from build123d import *

# Parameters (mm, degrees)
F0_W      = 100
F0_H      = 70
F1_DEPTH  = 60
F3_DEPTH  = 70.001
F4_R      = 2
F5_DEPTH  = 60.001
F6_R      = 28.75
F7_DEPTH  = 60.001
F8_T      = -2.54
F9_R      = 31.29
F9_R_2    = 28.75
F9_R_3    = 4.54
F9_R_4    = 2
F10_DEPTH = 55
F11_W     = 8.9
F11_H     = 11
F12_DEPTH = 25.4


with BuildPart() as f1:
    # F0 (on Top) → F1 (new body)
    with BuildSketch(Plane.XY):
        Rectangle(F0_W, F0_H)
    extrude(amount=F1_DEPTH)

    # F2 (on face) → F3 (cut, through all)
    with BuildSketch(Plane.XZ.offset(35)):
        Polygon((-50, 60), (-50, 0), (-29.1, 60), align=None)
        Polygon((30.9, 60), (50, 0), (50, 60), align=None)
    extrude(amount=-F3_DEPTH, mode=Mode.SUBTRACT)

    # F4 (on face) → F5 (cut, through all)
    with BuildSketch(Plane.XY.offset(60)):
        with Locations((-24.7, 25.507)):
            Circle(F4_R)
        with Locations((26.5, 25.507)):
            Circle(F4_R)
        with Locations((26.5, -25.493)):
            Circle(F4_R)
        with Locations((-24.7, -25.493)):
            Circle(F4_R)
    extrude(amount=-F5_DEPTH, mode=Mode.SUBTRACT)

    # F6 (on face) → F7 (cut, through all)
    with BuildSketch(Plane.XY.offset(60)):
        with Locations((0.92, 0)):
            Circle(F6_R)
    extrude(amount=-F7_DEPTH, mode=Mode.SUBTRACT)

    # F8
    f8_openings = [f1.faces().sort_by_distance(p)[0] for p in [
        (0, 33.779344, 0),
    ]]
    offset(amount=F8_T, openings=f8_openings)

    # F9 (on face) → F10 (cut)
    with BuildSketch(Plane(origin=(0, 0, 0), x_dir=(1, 0, 0), z_dir=(0, 0, -1))):
        with Locations((0.92, 0)):
            Circle(F9_R)
        with Locations((0.92, 0)):
            Circle(F9_R_2, mode=Mode.SUBTRACT)
        with Locations((-24.7, 25.493)):
            Circle(F9_R_3)
        with Locations((-24.7, 25.493)):
            Circle(F9_R_4, mode=Mode.SUBTRACT)
        with Locations((26.5, 25.493)):
            Circle(F9_R_3)
        with Locations((26.5, 25.493)):
            Circle(F9_R_4, mode=Mode.SUBTRACT)
        with Locations((26.5, -25.507)):
            Circle(F9_R_3)
        with Locations((26.5, -25.507)):
            Circle(F9_R_4, mode=Mode.SUBTRACT)
        with Locations((-24.7, -25.507)):
            Circle(F9_R_3)
        with Locations((-24.7, -25.507)):
            Circle(F9_R_4, mode=Mode.SUBTRACT)
    extrude(amount=-F10_DEPTH, mode=Mode.SUBTRACT)

    # F11 (on face) → F12 (cut)
    with BuildSketch(Plane(origin=(0, 35, 0), x_dir=(-1, 0, 0), z_dir=(0, 1, 0))):
        with Locations((0.05, 5.5)):
            Rectangle(F11_W, F11_H)
    extrude(amount=-F12_DEPTH, mode=Mode.SUBTRACT)


solid = f1.part
Geometry: final body of the model. Coordinates: model frame, mm. A direction names the side the tool comes from. Give positions to 0.01 mm unless a question says otherwise; leave off trailing zeros. Write each loop counter-clockwise with the first axis right and the second up, starting at its lowest first coordinate (ties: lowest second). Pieces come first, ordered by that corner, then holes. Notation, with made-up numbers: (89.5, 4.5) - (134.5, 4.5) arc R19 cw to (134.5, 18.5) - close; hole circle Ø1 at (73.5, -4.5). An arc over 180 degrees is marked (long way). Return JSON: item names as keys, results as strings. Group by question number.
1) Section C-C on z = 41. Return the cut outline in (x, y), plus the area to 3 significant figures.
2) First-contact query: P1, Ø10, axis at x = 25, y = -25, coming from the -Z side; P2, Ø5, axis at y = -8.5, z = 11, coming from the -X side; P3, Ø3, axis at y = -23.5, z = 46.5, coming from the -X side (3 decimals). Flat tips, straight axial feed; report the tip coordinate or a pass-through.
3) Section A-A on y = 0. Return the cut outline in (x, z).
4) Section B-B on x = 0.92. Return the cut outline in (y, z), plus the area to 3 significant figures.
5) Line query: line 1 (Y direction, x = -12.5, z = 8.5); line 2 (Y direction, x = 0.92, z = 57.75); line 3 (X direction, y = 6, z = 24). Output: solid intervals per line, ascending.
6) Section D-D on x = -24.7. State how many separate pieces and enclosed holes the cut face has, plus the area to 3 significant figures.
7) Set-up query: faces 1 (the flat face through (29, 9, 55)), 2 (the flat face through (-4.5, 34, 5)), 3 (the cylindrical face through (-26.7, 25.59, 57.54)). Return all of +Z, -Z, +X, -X, +Y, -Y with unobstructed straight access to the full face (end or side cutting, diameter ignored); none if empty.
Filled in:
{
 "1": {"outline": "(-35.72, -35) - (36.95, -35) - (36.95, 35) - (-35.72, 35) - close; hole (-33.03, -32.46) - (34.28, -32.46) - (34.28, 32.46) - (-33.03, 32.46) - close", "area": "717 mm^2"},
 "2": {"P1": "stops at z = 55", "P2": "stops at x = -47.04", "P3": "stops at x = -34.325"},
 "3": {"outline": "(-50, 0) - (-47.31, 0) - (-30.37, 48.63) - (-30.37, 55) - (-27.83, 55) - (-27.83, 60) - (-29.1, 60) - close; (29.67, 55) - (32.21, 55) - (32.21, 47.51) - (47.33, 0) - (50, 0) - (30.9, 60) - (29.67, 60) - close"},
 "4": {"outline": "(-35, 0) - (-32.46, 0) - (-32.46, 57.46) - (-31.29, 57.46) - (-31.29, 55) - (-28.75, 55) - (-28.75, 60) - (-35, 60) - close; (28.75, 55) - (31.29, 55) - (31.29, 57.46) - (32.46, 57.46) - (32.46, 11) - (35, 11) - (35, 60) - (28.75, 60) - close", "area": "308 mm^2"},
 "5": {"line 1": "y = -35 to -32.46, 32.46 to 35", "line 2": "y = -35 to -28.75, 28.75 to 35", "line 3": "x = -41.64 to -38.95, 39.69 to 42.36"},
 "6": {"separate pieces": "4", "enclosed holes": "0", "area": "432 mm^2"},
 "7": {"face 1": "-Z", "face 2": "-Z, +Y", "face 3": "+Z, -Z"}
}
